Input: part model. Units: mm. Frame: model coordinates. A direction names the side the tool comes from. Round coordinates to 2 decimals unless told otherwise and drop trailing zeros. Loops run counter-clockwise (first coordinate to the right, second up) from the corner with the lowest first, then second, coordinate; pieces in that order, holes last.
(1) Line query: line 1 (Y direction, x = 1.95, z = 1.1); line 2 (Y direction, x = 46.2, z = 0.8); line 3 (X direction, y = 1.75, z = 0.55). Output: solid intervals per line, ascending.
(2) Access query for faces 4 (the face through (6, 13, 3)), 5 (the face through (3, 16.6, 3)), 6 (the face through (3, 9, 3)). Directions: +Z, -Z, +X, -X, +Y, -Y. A direction counts if a zero-diameter tool reaches every point of the face in a straight line with its end or side. Return the directions, or none.
(3) Cut plane B-B, the plane y = 13.5. Output: boundary loops of the cut face in (x, z).
(4) Draft query along Y for faces 1 (the face through (44.85, 2.21, 0.74)), 2 (the face through (24, 0, 1)), 3 (the face through (48.15, 13, 1)). Return one class per face: released by +Y, released by -Y, zero draft, split by the parting line, or undercut.
(5) Cut plane C-C, the plane x = 36. Output: boundary loops of the cut face in (y, z).
(6) Cut plane A-A, the plane z = 0.75. Output: boundary loops of the cut face in (x, y).
(7) First-contact query: pin 1 Ø1 at (y, z) = (4, 3) entering from +X; pin 2 Ø8 at (x, y) = (6.5, 3) entering from +Z; pin 3 Ø2 at (y, z) = (14.5, 3) entering from +X; pin 4 Ø0.8 at (x, z) = (3, 2.5) entering from +Y. Flat tips, straight axial feed; report the tip coordinate or a pass-through.
(8) Cut plane D-D, the plane z = 3.2. Output: boundary loops of the cut face in (x, y).
from build123d import *

# Parameters (mm, degrees)
F0_R     = 1.35
F1_DEPTH = 1.5
F2_W     = 6
F2_H     = 7.6
F3_DEPTH = 2.5


with BuildPart() as f1:
    # F0 (on Top) → F1 (new body)
    with BuildSketch(Plane.XY):
        with BuildLine():
            ThreePointArc((0, 2), (0.585786, 0.585786), (2, 0))
            Line((2, 0), (46.15, 0))
            ThreePointArc((46.15, 0), (47.564214, 0.585786), (48.15, 2))
            Line((48.15, 2), (48.15, 23.6))
            ThreePointArc((48.15, 23.6), (47.564214, 25.014214), (46.15, 25.6))
            Line((46.15, 25.6), (2, 25.6))
            ThreePointArc((2, 25.6), (0.585786, 25.014214), (0, 23.6))
            Line((0, 23.6), (0, 2))
        make_face()
        with Locations((1.95, 2.15)):
            Circle(F0_R, mode=Mode.SUBTRACT)
        with Locations((46.2, 2.15)):
            Circle(F0_R, mode=Mode.SUBTRACT)
        with Locations((1.95, 23.45)):
            Circle(F0_R, mode=Mode.SUBTRACT)
        with Locations((46.2, 23.6)):
            Circle(F0_R, mode=Mode.SUBTRACT)
    extrude(amount=F1_DEPTH)

    # F2 (on face) → F3 (join)
    with BuildSketch(Plane.XY.offset(1.5)):
        with Locations((3, 12.8)):
            Rectangle(F2_W, F2_H)
    extrude(amount=F3_DEPTH)


solid = f1.part
Reported:
1. line 1: y = 0 to 0.8, 3.5 to 22.1, 24.8 to 25.6
1. line 2: y = 0 to 0.8, 3.5 to 22.25, 24.95 to 25.6
1. line 3: x = 0.02 to 0.66, 3.24 to 44.91, 47.49 to 48.13
2. face 4: +Z, +X, +Y, -Y
2. face 5: +Z, +X, -X, +Y
2. face 6: +Z, +X, -X, -Y
3. outline: (0, 0) - (48.15, 0) - (48.15, 1.5) - (6, 1.5) - (6, 4) - (0, 4) - close
4. face 1: undercut
4. face 2: released by -Y
4. face 3: zero draft
5. outline: (0, 0) - (25.6, 0) - (25.6, 1.5) - (0, 1.5) - close
6. outline: (0, 2) arc R2 ccw to (2, 0) - (46.15, 0) arc R2 ccw to (48.15, 2) - (48.15, 23.6) arc R2 ccw to (46.15, 25.6) - (2, 25.6) arc R2 ccw to (0, 23.6) - close; hole circle Ø2.7 at (1.95, 2.15); hole circle Ø2.7 at (1.95, 23.45); hole circle Ø2.7 at (46.2, 2.15); hole circle Ø2.7 at (46.2, 23.6)
7. pin 1: passes through
7. pin 2: stops at z = 1.5
7. pin 3: stops at x = 6
7. pin 4: stops at y = 16.6
8. outline: (0, 9) - (6, 9) - (6, 16.6) - (0, 16.6) - close
